```python
from build123d import *

# Parameters (mm, degrees)
F1_DEPTH = 33.9
F2_R     = 1
F4_W     = 15.65184
F4_H     = 26.75
F5_DEPTH = 33.1


with BuildPart() as f1:
    # F0 (on Top) → F1 (new body)
    with BuildSketch(Plane.XY):
        with BuildLine():
            Line((7.841366, 7.324094), (22.777264, 7.324094))
            Line((22.777264, 7.324094), (22.777264, -19.425906))
            Line((22.777264, -19.425906), (7.841366, -19.425906))
            ThreePointArc((7.841366, -19.425906), (4.377264, -17.425906), (0.913162, -19.425906))
            Line((0.913162, -19.425906), (-11.222736, -19.425906))
            Line((-11.222736, -19.425906), (-11.222736, -14.225906))
            Line((-11.222736, -14.225906), (-16.422736, -14.225906))
            Line((-16.422736, -14.225906), (-16.422736, -19.425906))
            Line((-16.422736, -19.425906), (-27.022736, -19.425906))
            Line((-27.022736, -19.425906), (-27.022736, -8.650906))
            Line((-27.022736, -8.650906), (-32.222736, -8.650906))
            Line((-32.222736, -8.650906), (-32.222736, -19.625906))
            ThreePointArc((-32.222736, -19.625906), (-30.75827, -23.16144), (-27.222736, -24.625906))
            Line((-27.222736, -24.625906), (24.777264, -24.625906))
            ThreePointArc((24.777264, -24.625906), (28.312798, -23.16144), (29.777264, -19.625906))
            Line((29.777264, -19.625906), (29.777264, 7.524094))
            ThreePointArc((29.777264, 7.524094), (28.312798, 11.059628), (24.777264, 12.524094))
            Line((24.777264, 12.524094), (-27.222736, 12.524094))
            ThreePointArc((-27.222736, 12.524094), (-30.75827, 11.059628), (-32.222736, 7.524094))
            Line((-32.222736, 7.524094), (-32.222736, -3.450906))
            Line((-32.222736, -3.450906), (-27.022736, -3.450906))
            Line((-27.022736, -3.450906), (-27.022736, 7.324094))
            Line((-27.022736, 7.324094), (-16.422736, 7.324094))
            Line((-16.422736, 7.324094), (-16.422736, 2.124094))
            Line((-16.422736, 2.124094), (-11.222736, 2.124094))
            Line((-11.222736, 2.124094), (-11.222736, 7.324094))
            Line((-11.222736, 7.324094), (0.913162, 7.324094))
            ThreePointArc((0.913162, 7.324094), (4.377264, 5.324094), (7.841366, 7.324094))
        make_face()
    extrude(amount=F1_DEPTH)

    # F2
    f2_edges = [f1.edges().sort_by_distance(p)[0] for p in [
        (-16.422736, -14.225906, 16.95),
        (-11.222736, -14.225906, 16.95),
        (-11.222736, 2.124094, 16.95),
        (-16.422736, 2.124094, 16.95),
        (-27.022736, -8.650906, 16.95),
        (-32.222736, -8.650906, 16.95),
        (-27.022736, -3.450906, 16.95),
        (-32.222736, -3.450906, 16.95),
    ]]
    fillet(f2_edges, radius=F2_R)

    # F4 (on face) → F5 (cut)
    with BuildSketch(Plane(origin=(0.897894, 0, 5.092212), x_dir=(0.984808, 0, -0.173648), z_dir=(-0.173648, 0, -0.984808))):
        with Locations((3.283218, 6.050906)):
            Rectangle(F4_W, F4_H)
    extrude(amount=-F5_DEPTH, mode=Mode.SUBTRACT)


solid = f1.part
```
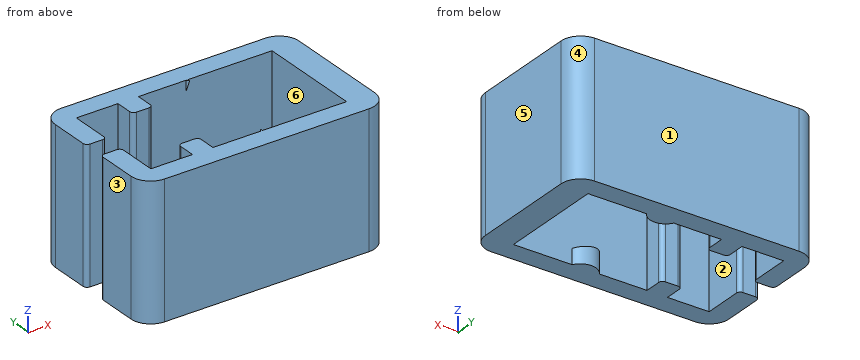
Design review of the part built by this model. Coordinates are the model's own, in mm. Face numbers are marked on the shaded views. A direction names the side the tool comes from. Round coordinates to 2 decimals unless told otherwise and drop trailing zeros. Write each loop counter-clockwise with the first axis right and the second up, starting at its lowest first coordinate (ties: lowest second). Pieces come first, ordered by that corner, then holes.
Item 1: We need section A-A on x = -2.5. Write out the cut boundary in (y, z), and give its area (3 significant figures).
Item 2: For probe 1 along X at (y, z) = (6.5, 32); probe 2 along Y at (x, z) = (-18, 15); probe 3 along X at (y, z) = (-12, 32), list the stretches that pass through material, from the lowest coordinate up.
Item 3: Clearance check with flat-ended pins moving along their axes: pin 1 Ø12 at (x, y) = (-22.5, -16.5) entering from -Z; pin 2 Ø1 at (x, z) = (-30.5, 21) entering from +Y. State where each tip first meets the part, or that it passes through.
Item 4: For the marked faces 5 and 6, list the 3-axis set-ups (+Z, -Z, +X, -X, +Y, -Y) from which the entire face can be reached by the end or side of a thin tool; tool diameter is ignored.
Item 5: We need section B-B on y = -0.5. Write out the cut boundary in (x, z).
Item 6: The part is to be moulded in two halves that separate along X. For the marked faces 1, 2, 3 and 4, say which applies: +X half, -X half, draft (parallel to the pull), parting line (faces both ways), or undercut.
Returned:
1. outline: (-24.63, 0) - (-19.43, 0) - (-19.43, 33.9) - (-24.63, 33.9) - close; (7.32, 0) - (12.52, 0) - (12.52, 33.9) - (7.32, 33.9) - close
1. area: 353 mm2
2. probe 1: x = -32.22 to -27.02, -16.42 to -11.22, 22.78 to 29.78
2. probe 2: y = -24.63 to -19.43, 7.32 to 12.52
2. probe 3: x = -32.22 to -27.02, 22.78 to 29.78
3. pin 1: stops at z = 0
3. pin 2: stops at y = 11.68
4. face 5: +Z, -Z, +X, +Y, -Y
4. face 6: +Z, -Z
5. outline: (-32.22, 0) - (-27.02, 0) - (-27.02, 33.9) - (-32.22, 33.9) - close; (22.78, 0) - (29.78, 0) - (29.78, 33.9) - (22.78, 33.9) - close
6. face 1: draft
6. face 2: undercut
6. face 3: -X half
6. face 4: +X half
